Geometry: final body of the model. Coordinates: model frame, mm. A direction names the side the tool comes from. Round coordinates to 2 decimals unless told otherwise and drop trailing zeros. Loops run counter-clockwise (first coordinate to the right, second up) from the corner with the lowest first, then second, coordinate; pieces in that order, holes last. Notation, with made-up numbers: (-15, -21.5) -> (31, -21.5) arc R28 ccw to (31, 5.5) -> close; hole circle Ø9 at (65, 27.25). An arc over 180 degrees is marked (long way). Answer in a Markdown table with one row per item.
```python
from build123d import *

# Parameters (mm, degrees)
SKETCH1_W           = 131.7625
SKETCH1_H           = 184.15
BOSS_EXTRUDE1_DEPTH = 196.85
SKETCH2_W           = 7.243123939
SKETCH2_H           = 8.967677257
SKETCH2_H_2         = 9.31258792
BOSS_EXTRUDE2_DEPTH = 10.16


with BuildPart() as part:
    # Sketch1 → Boss-Extrude1 (new body)
    with BuildSketch(Plane(origin=(0, 0, 0), x_dir=(1, 0, 0), z_dir=(0, 1, 0))):
        with Locations((-65.88125, -92.075)):
            Rectangle(SKETCH1_W, SKETCH1_H)
    extrude(amount=BOSS_EXTRUDE1_DEPTH)


with BuildPart() as part_1:
    # Body-Move/Copy1: moved
    add(part.part.moved(Location((118.999, -260.35, -108.458))))

    # Sketch2 → Boss-Extrude2 (add)
    with BuildSketch(Plane.XY.offset(75.692)):
        with Locations((-0.518268716, -71.195276502)):
            Rectangle(SKETCH2_W, SKETCH2_H)
        with Locations((-0.518268716, -251.756008966)):
            Rectangle(SKETCH2_W, SKETCH2_H_2)
    extrude(amount=BOSS_EXTRUDE2_DEPTH)


solid = part_1.part
```
Item 1: Line query: probe 1 along Z at (x, y) = (8, -241). Output: solid intervals per line, ascending. Write a range as [from, to].
Answer:
| item | result |
|---|---|
| probe 1 | z = [-108.46, 75.69] |
Item 2: Pin query (flat end, axial travel): pin 1 Ø7.5 at (y, z) = (-251, 81) entering from +X; pin 2 Ø8 at (x, z) = (-2, 82.5) entering from +Y; pin 3 Ø10 at (x, y) = (20, -222.5) entering from +Z. Return the tip coordinate at first contact, or that it passes through.
Answer:
| item | result |
|---|---|
| pin 1 | stops at x = 3.1 |
| pin 2 | stops at y = -66.71 |
| pin 3 | stops at z = 75.69 |
Item 3: Draft query along Y for faces 1 (the face through (-1, -247.1, 81)), 2 (the face through (52, -163, -108.458)), 3 (the face through (52, -260.35, -18)). Return one class per face: pulls with the +Y half, pulls with the -Y half, needs draft (parallel to the pull), parting line crosses it, or undercut.
Answer:
| item | result |
|---|---|
| face 1 | undercut |
| face 2 | needs draft |
| face 3 | pulls with the -Y half |
Item 4: Cut plane B-B (x = 7). Output: boundary loops of the cut face in (y, z), then the cut area to 4 significant figures.
Answer:
| item | result |
|---|---|
| outline | (-260.35, -108.46) -> (-63.5, -108.46) -> (-63.5, 75.69) -> (-260.35, 75.69) -> close |
| area | 36,250 mm² |
Item 5: Cut plane A-A (y = -109.5). Output: boundary loops of the cut face in (x, z).
Answer:
| item | result |
|---|---|
| outline | (-12.76, -108.46) -> (119, -108.46) -> (119, 75.69) -> (-12.76, 75.69) -> close |
Item 6: Reachability of faces 4 (the face through (-1, -75.679, 81)), 5 (the face through (3.103, -252, 81)), 6 (the face through (-1, -256.412, 81)) from +Z, -Z, +X, -X, +Y, -Y: full face, straight path, thin tool, end or side. Return the list, or none.
Answer:
| item | result |
|---|---|
| face 4 | +Z, +X, -X |
| face 5 | +Z, +X, +Y, -Y |
| face 6 | +Z, +X, -X, -Y |
